```python
from build123d import *

# Parameters (mm, degrees)
F1_R     = 12.5
F1_R_2   = 10.5
F2_DEPTH = 20
F3_R     = 10.75
F4_DEPTH = 10
F5_R     = 0.5


with BuildPart() as f2:
    # F1 (on offset) → F2 (new body)
    with BuildSketch(Plane.XY.offset(36.5)):
        Circle(F1_R)
        Circle(F1_R_2, mode=Mode.SUBTRACT)
    extrude(amount=F2_DEPTH)

    # F3 (on face) → F4 (cut)
    with BuildSketch(Plane.XY.offset(56.5)):
        Circle(F3_R)
    extrude(amount=-F4_DEPTH, mode=Mode.SUBTRACT)

    # F5
    f5_edges = [f2.edges().sort_by_distance(p)[0] for p in [
        (-10.75, 0, 56.5),
        (-10.5, 0, 36.5),
    ]]
    fillet(f5_edges, radius=F5_R)


solid = f2.part
```
Design review of the part built by this model. Coordinates are the model's own, in mm. A direction names the side the tool comes from. Coordinates: 2 decimals unless noted, no trailing zeros. Order: outer loops, then holes, each group sorted by start corner. A loop starts at its lowest first (then second) coordinate and runs counter-clockwise, first axis right, second up.
1) Take a section at C-C, the plane z = 46. Give the boundary of the cut face in (x, y).
2) Take a section at D-D, the plane z = 54. Give the boundary of the cut face in (x, y), and give its area (3 significant figures).
3) Clearance check with flat-ended pins moving along their axes: pin 1 (5 mm diameter, centred on x = -5, z = 40.5, fed in from -Y); pin 2 (1.5 mm diameter, centred on y = -8, z = 53, fed in from +X); pin 3 (2 mm diameter, centred on x = -8, z = 48, fed in from +Y). State where each tip first meets the part, or that it passes through.
4) For faces 1 (the cylindrical face through (11.923, 3.755, 46.36)), 2 (the cylindrical face through (-1.4, 10.66, 51.32)), list the 3-axis set-ups (+Z, -Z, +X, -X, +Y, -Y) from which the entire face can be reached by the end or side of a thin tool; tool diameter is ignored.
5) Take a section at A-A, the plane x = 0. Give the boundary of the cut face in (y, z).
6) Wall thickness on line 1 along Y through (x, z) = (0.25, 39); line 2 along Y through (x, z) = (0, 49.75); line 3 along X through (y, z) = (-8, 46.25): over which ranges is each line inside the solid? List them lowest first.
Returned:
1. outline: circle Ø25 at (0, 0); hole circle Ø21 at (0, 0)
2. outline: circle Ø25 at (0, 0); hole circle Ø21.5 at (0, 0)
2. area: 128 mm2
3. pin 1: stops at y = -12.25
3. pin 2: stops at x = 10.18
3. pin 3: stops at y = 10.36
4. face 1: +Z, -Z
4. face 2: +Z
5. outline: (-12.5, 36.5) - (-11, 36.5) arc R0.5 ccw to (-10.5, 37) - (-10.5, 46.5) - (-10.75, 46.5) - (-10.75, 56) arc R0.5 ccw to (-11.25, 56.5) - (-12.5, 56.5) - close; (10.5, 37) arc R0.5 ccw to (11, 36.5) - (12.5, 36.5) - (12.5, 56.5) - (11.25, 56.5) arc R0.5 ccw to (10.75, 56) - (10.75, 46.5) - (10.5, 46.5) - close
6. line 1: y = -12.5 to -10.5, 10.5 to 12.5
6. line 2: y = -12.5 to -10.75, 10.75 to 12.5
6. line 3: x = -9.6 to -6.8, 6.8 to 9.6
